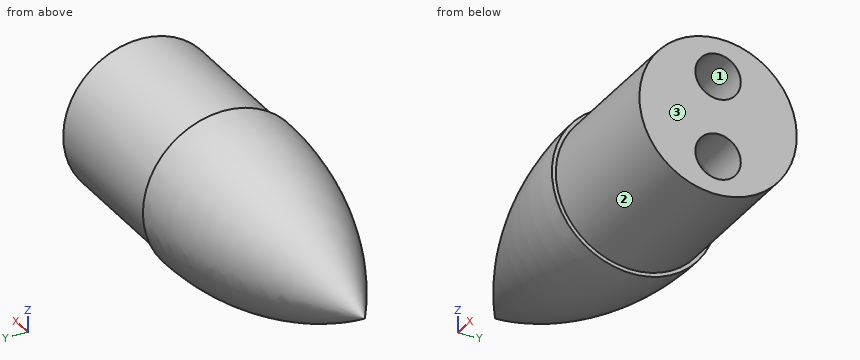
```python
from build123d import *

# Parameters (mm, degrees)
SKETCH2_R           = 37.846
BOSS_EXTRUDE1_DEPTH = 50.8
SKETCH3_R           = 10.922
SKETCH4_R           = 37.846
SKETCH4_R_2         = 10.922
BOSS_EXTRUDE2_DEPTH = 25.4


with BuildPart() as part:
    # Sketch1 → Revolve1 (revolve)
    with BuildSketch(Plane.XY):
        with BuildLine():
            Line((126.999999998, 0), (126.999999998, 39.712900001))
            add(Edge.make_bspline(
                [(-1e-09, 0), (63.499999999, 39.7129), (126.999999998, 39.712900001)],
                knots=[0.074879484, 0.074879484, 0.074879484, 0.915898135, 0.915898135, 0.915898135], degree=2))
            Line((-1e-09, 0), (126.999999998, 0))
        make_face()
    revolve(axis=Axis((-1e-09, 0, 0), (1, 0, 0)))

    # Sketch2 → Boss-Extrude1 (add)
    with BuildSketch(Plane(origin=(126.999999998, 0, 0), x_dir=(0, 0, -1), z_dir=(1, 0, 0))):
        with Locations(Location((0, 0, 0), (0, 0, 180))):
            Circle(SKETCH2_R)
    extrude(amount=BOSS_EXTRUDE1_DEPTH)

    # Sketch3 → Cut-Revolve1 (revolve, cut)
    with BuildSketch(Plane(origin=(177.799999998, 0, 0), x_dir=(0, 0, -1), z_dir=(1, 0, 0)), mode=Mode.PRIVATE) as cut_revolve1_sk:
        with Locations((-19.347570256, 0)):
            Circle(SKETCH3_R)
    revolve(cut_revolve1_sk.sketch.rotate(Axis((177.799999998, 0, 0), (0, 1, 0)), 270), axis=Axis((177.799999998, 0, 0), (0, 1, 0)), mode=Mode.SUBTRACT)

    # Sketch4 → Boss-Extrude2 (add)
    with BuildSketch(Plane(origin=(177.799999998, 0, 0), x_dir=(0, 0, -1), z_dir=(1, 0, 0))):
        with Locations(Location((0, 0, 0), (0, 0, 180))):
            Circle(SKETCH4_R)
        with Locations(Location((-19.347570256, 0, 0), (0, 0, 180))):
            Circle(SKETCH4_R_2, mode=Mode.SUBTRACT)
        with Locations((19.347570256, 0)):
            Circle(SKETCH4_R_2, mode=Mode.SUBTRACT)
    extrude(amount=BOSS_EXTRUDE2_DEPTH)


solid = part.part
```
For this review, take the finished solid that the model builds, in its own axes (mm). Face numbers are marked on the shaded views. Give positions to 0.01 mm unless a question says otherwise; leave off trailing zeros. Answer as a JSON object with one key per item and string values. Group by question number.
Item 1: For pin 1 Ø4 at (x, y) = (97.5, -24.5) entering from -Z; pin 2 Ø3 at (x, z) = (65, 26) entering from +Y; pin 3 Ø2 at (x, y) = (143, -24.5) entering from -Z, all flat-tipped, find the tip position at first contact; note any pin that passes through.
Item 2: Draft analysis for pull direction Y (two halves, no side actions). For the marked faces 1, 2 and 3, state which applies: +Y half, -Y half, draft (parallel to the pull), parting line (faces both ways), or undercut.
Item 3: For probe 1 along Z at (x, y) = (175.5, 1); probe 2 along Y at (x, z) = (185, -17); probe 3 along Y at (x, z) = (165.5, 4), list the stretches that pass through material, from the lowest coordinate up. Write a range as [from, to].
Check result:
{
 "1": {"pin 1": "stops at z = -30.13", "pin 2": "stops at y = 17.88", "pin 3": "stops at z = -29.67"},
 "2": {"face 1": "undercut", "face 2": "parting line", "face 3": "draft"},
 "3": {"probe 1": "z = [-37.83, -30.14], [-8.15, 8.15], [30.14, 37.83]", "probe 2": "y = [-33.81, -10.67], [10.67, 33.81]", "probe 3": "y = [-37.63, -8.84], [8.84, 37.63]"}
}
